```python
from build123d import *

# Parameters (mm, degrees)
SKETCH_1_W          = 70
SKETCH_1_H          = 60
EXTRUDE_1_DEPTH     = 3
SKETCH_2_R          = 1.5
CUT_EXTRUDE_1_DEPTH = 93.244241013
FILLET_1_R          = 3


with BuildPart() as part:
    # 草图1 → 凸台-拉伸1 (new body)
    with BuildSketch(Plane(origin=(0, 0, 0), x_dir=(1, 0, 0), z_dir=(0, 1, 0))):
        with Locations((35, -30)):
            Rectangle(SKETCH_1_W, SKETCH_1_H)
    extrude(amount=EXTRUDE_1_DEPTH)

    # 草图2 → 切除-拉伸1 (cut, through all)
    with BuildSketch(Plane(origin=(0, 3, 0), x_dir=(1, 0, 0), z_dir=(0, 1, 0))):
        with Locations(Location((57, -5, 0), (0, 0, 270))):
            Circle(SKETCH_2_R)
        with Locations(Location((41, -5, 0), (0, 0, 270))):
            Circle(SKETCH_2_R)
        with Locations(Location((57, -55, 0), (0, 0, 270))):
            Circle(SKETCH_2_R)
        with Locations(Location((41, -55, 0), (0, 0, 270))):
            Circle(SKETCH_2_R)
    extrude(amount=-CUT_EXTRUDE_1_DEPTH, mode=Mode.SUBTRACT)

    # 圆角1
    fillet_1_edges = [part.edges().sort_by_distance(p)[0] for p in [
        (0, 1.5, 0),
        (70, 1.5, 0),
        (70, 1.5, 60),
        (0, 1.5, 60),
    ]]
    fillet(fillet_1_edges, radius=FILLET_1_R)


solid = part.part
```
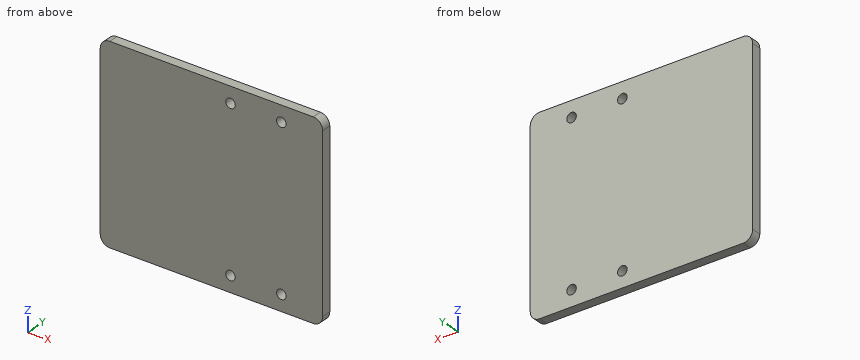
Part model, mm, in its own coordinate system. Round coordinates to 2 decimals unless told otherwise and drop trailing zeros. Write each loop counter-clockwise with the first axis right and the second up, starting at its lowest first coordinate (ties: lowest second). Pieces come first, ordered by that corner, then holes.
Item 1: Cut at A-A, the plane z = 55. Give the cut face in (x, y).
Results:
outline: (0, 0) - (39.5, 0) - (39.5, 3) - (0, 3) - close; (42.5, 0) - (55.5, 0) - (55.5, 3) - (42.5, 3) - close; (58.5, 0) - (70, 0) - (70, 3) - (58.5, 3) - close
Item 2: Cut at B-B, the plane x = 57. Give the cut face in (y, z).
Results:
outline: (0, 0) - (3, 0) - (3, 3.5) - (0, 3.5) - close; (0, 6.5) - (3, 6.5) - (3, 53.5) - (0, 53.5) - close; (0, 56.5) - (3, 56.5) - (3, 60) - (0, 60) - close
Item 3: Probe L1, parallel to X at y = 0.9, z = 5; L2, parallel to X at y = 0.4, z = 54; L3, parallel to Z at x = 42, y = 0.5. List the from-to ranges inside material, lowest first.
Results:
L1: x = 0 to 39.5, 42.5 to 55.5, 58.5 to 70
L2: x = 0 to 39.88, 42.12 to 55.88, 58.12 to 70
L3: z = 0 to 3.88, 6.12 to 53.88, 56.12 to 60
